```python
from build123d import *

# Parameters (mm, degrees)
BOSS_EXTRUDE4_DEPTH      = 20
SKETCH3_R                = 8.25
CUT_EXTRUDE1_DEPTH       = 7
CUT_EXTRUDE2_START       = -7
SKETCH4_R                = 8.25
CUT_EXTRUDE2_DEPTH       = 7
CUT_EXTRUDE3_DEPTH       = 128.220772675
SKETCH6_R                = 5
CUT_EXTRUDE4_DEPTH       = 16.6
FILLET1_R                = 3
BOSS_EXTRUDE5_DEPTH      = 20
BOSS_EXTRUDE6_DEPTH      = 46
BOSS_EXTRUDE6_DEPTH_BACK = 25
SKETCH8_R                = 11
SKETCH8_R_2              = 8.25
BOSS_EXTRUDE7_REACH      = 138.572
SKETCH9_W                = 20
SKETCH9_H                = 10
FILLET2_R                = 5
FILLET5_R                = 5
SKETCH10_W               = 60.25
SKETCH10_H               = 70.5
CUT_EXTRUDE5_DEPTH       = 128.619062056
BOSS_EXTRUDE8_DEPTH      = 20
BOSS_EXTRUDE9_START      = -20
SKETCH12_R               = 11
BOSS_EXTRUDE9_DEPTH      = 20
SKETCH13_OUTSIDE_W       = 202.602
SKETCH13_OUTSIDE_H       = 60.102
SKETCH13_OUTSIDE_W_2     = 164.5
SKETCH13_OUTSIDE_H_2     = 20
CUT_EXTRUDE6_DEPTH       = 152.565373684


with BuildPart() as part:
    # Sketch2 → Boss-Extrude4 (new body)
    with BuildSketch(Plane.XY):
        with BuildLine():
            Line((-100, 10.25), (0, 10.25))
            ThreePointArc((0, 10.25), (10.25, 0), (0, -10.25))
            Line((0, -10.25), (-100, -10.25))
            ThreePointArc((-100, -10.25), (-110.25, 0), (-100, 10.25))
        make_face()
        with BuildLine():
            Line((-7.247844507, -7.247844507), (-57.247844507, 42.752155493))
            ThreePointArc((-57.247844507, 42.752155493), (-57.247844507, 57.247844507), (-42.752155493, 57.247844507))
            Line((-42.752155493, 57.247844507), (7.247844507, 7.247844507))
            ThreePointArc((7.247844507, 7.247844507), (7.247844507, -7.247844507), (-7.247844507, -7.247844507))
        make_face()
        with BuildLine():
            Line((-107.247844507, 7.247844507), (-57.247844507, 57.247844507))
            ThreePointArc((-57.247844507, 57.247844507), (-42.752155493, 57.247844507), (-42.752155493, 42.752155493))
            Line((-42.752155493, 42.752155493), (-92.752155493, -7.247844507))
            ThreePointArc((-92.752155493, -7.247844507), (-107.247844507, -7.247844507), (-107.247844507, 7.247844507))
        make_face()
    extrude(amount=BOSS_EXTRUDE4_DEPTH)

    # Sketch3 → Cut-Extrude1 (cut)
    with BuildSketch(Plane(origin=(0, 0, 0), x_dir=(-1, 0, 0), z_dir=(0, 0, -1))):
        Circle(SKETCH3_R)
        with Locations((50, 50)):
            Circle(SKETCH3_R)
        with Locations((100, 0)):
            Circle(SKETCH3_R)
    extrude(amount=-CUT_EXTRUDE1_DEPTH, mode=Mode.SUBTRACT)

    # Sketch4 → Cut-Extrude2 (cut)
    with BuildSketch(Plane.XY.offset(20).offset(CUT_EXTRUDE2_START)):
        with Locations(Location((-100, 0, 0), (0, 0, 180))):
            Circle(SKETCH4_R)
        with Locations(Location((-50, 50, 0), (0, 0, 180))):
            Circle(SKETCH4_R)
        with Locations(Location((0, 0, 0), (0, 0, 180))):
            Circle(SKETCH4_R)
    extrude(amount=CUT_EXTRUDE2_DEPTH, mode=Mode.SUBTRACT)

    # Sketch5 → Cut-Extrude3 (cut, through all)
    with BuildSketch(Plane(origin=(0, 0, 0), x_dir=(-1, 0, 0), z_dir=(0, 0, -1))):
        Polygon((17.5, 8.25), (50, 40.75), (82.5, 8.25), align=None)
    extrude(amount=-CUT_EXTRUDE3_DEPTH, mode=Mode.SUBTRACT)

    # Sketch6 → Cut-Extrude4 (cut)
    with BuildSketch(Plane.XY.offset(20)):
        with Locations((-100, 0)):
            Circle(SKETCH6_R)
        with Locations((-50, 50)):
            Circle(SKETCH6_R)
        Circle(SKETCH6_R)
    extrude(amount=-CUT_EXTRUDE4_DEPTH, mode=Mode.SUBTRACT)

    # Fillet1
    fillet1_edges = [part.edges().sort_by_distance(p)[0] for p in [
        (-82.5, 8.25, 10),
        (-17.5, 8.25, 10),
        (-50, 40.75, 10),
    ]]
    fillet(fillet1_edges, radius=FILLET1_R)

    # Sketch7 → Boss-Extrude5 (add)
    with BuildSketch(Plane(origin=(0, 0, 0), x_dir=(-1, 0, 0), z_dir=(0, 0, -1))):
        with BuildLine():
            Line((-10.25, 14.75), (-10.25, 0))
            ThreePointArc((-10.25, 0), (-9.469765208, 3.922505182), (-7.247844507, 7.247844507))
            Line((-7.247844507, 7.247844507), (0.254310986, 14.75))
            Line((0.254310986, 14.75), (-10.25, 14.75))
        make_face()
        with BuildLine():
            Line((-10.25, -10.25), (0, -10.25))
            ThreePointArc((0, -10.25), (-7.247844507, -7.247844507), (-10.25, 0))
            Line((-10.25, 0), (-10.25, -10.25))
        make_face()
    extrude(amount=-BOSS_EXTRUDE5_DEPTH)

    # Sketch8 → Boss-Extrude6 (add, two sides: drawn at the far end of the back side and taken through both)
    # profile 1 of 3: a face of its own
    with BuildSketch(Plane(origin=(0, 14.75, 0), x_dir=(1, 0, 0), z_dir=(0, 1, 0)).offset(-BOSS_EXTRUDE6_DEPTH_BACK)):
        with BuildLine():
            Line((10.25, 0), (10.25, -10))
            ThreePointArc((10.25, -10), (13.110659193, -2.600599266), (20.204751131, 0.950226244))
            Line((20.204751131, 0.950226244), (10.25, 0))
        make_face()
    # profile 2 of 3: a face of its own
    with BuildSketch(Plane(origin=(0, 14.75, 0), x_dir=(1, 0, 0), z_dir=(0, 1, 0)).offset(-BOSS_EXTRUDE6_DEPTH_BACK)):
        with Locations((21.25, -10)):
            Circle(SKETCH8_R)
        with Locations(Location((21.25, -10, 0), (0, 0, 270))):
            Circle(SKETCH8_R_2, mode=Mode.SUBTRACT)
    # profile 3 of 3: a face of its own
    with BuildSketch(Plane(origin=(0, 14.75, 0), x_dir=(1, 0, 0), z_dir=(0, 1, 0)).offset(-BOSS_EXTRUDE6_DEPTH_BACK)):
        with BuildLine():
            Line((10.25, -10), (10.25, -20))
            Line((10.25, -20), (20.204751131, -20.950226244))
            ThreePointArc((20.204751131, -20.950226244), (13.110659193, -17.399400734), (10.25, -10))
        make_face()
    extrude(amount=BOSS_EXTRUDE6_DEPTH + BOSS_EXTRUDE6_DEPTH_BACK)

    # Boss-Extrude7: up to this plane
    boss_extrude7_end = Plane(origin=(7.247844507, 7.247844507, 20), z_dir=(-0.7071067811865439, -0.7071067811865512, 0))
    # Sketch9 → Boss-Extrude7 (add, up to the surface)
    with BuildSketch(Plane.ZY.offset(-10.25), mode=Mode.PRIVATE) as boss_extrude7_sk1:
        with Locations((10, 55.75)):
            Rectangle(SKETCH9_W, SKETCH9_H)
    boss_extrude7_tool1 = split(extrude(boss_extrude7_sk1.sketch, amount=BOSS_EXTRUDE7_REACH, mode=Mode.PRIVATE), bisect_by=boss_extrude7_end, keep=Keep.BOTH, mode=Mode.PRIVATE)
    add(boss_extrude7_tool1.solids().sort_by_distance((10.25, 55.75, 10))[0])

    # Fillet2
    # the kernel refuses this fillet: 5 mm, written as the material it adds along each edge
    with BuildSketch(Plane(origin=(10.25, 14.75, 0), x_dir=(-1, 0, 0), z_dir=(0, -1, 0)), Plane(origin=(10.25, -10.25, 20), x_dir=(-1, 0, 0), z_dir=(0, 1, 0))) as fillet2_piece_1:
        with BuildLine():
            CenterArc((FILLET2_R * 0.047619047619, FILLET2_R), FILLET2_R, 264.547378012, 5.452621988)
            Line((-FILLET2_R * 0.0474035768153, FILLET2_R * 0.00452488687783), (0, 0))
            Line((0, 0), (FILLET2_R * 0.047619047619, 0))
        make_face()
    extrude(amount=25)
    with BuildSketch(Plane(origin=(10.25, 50.75, 0), x_dir=(-1, 0, 0), z_dir=(0, 1, 0)), Plane(origin=(10.25, 60.75, 20), x_dir=(-1, 0, 0), z_dir=(0, -1, 0))) as fillet2_piece_2:
        with BuildLine():
            CenterArc((FILLET2_R * 0.047619047619, -FILLET2_R), FILLET2_R, 90, 5.452621988)
            Line((-FILLET2_R * 0.0474035768153, -FILLET2_R * 0.00452488687783), (0, 0))
            Line((0, 0), (FILLET2_R * 0.047619047619, 0))
        make_face()
    extrude(amount=10)

    # Fillet5
    fillet5_edges = [part.edges().sort_by_distance(p)[0] for p in [
        (-0.254310986, 14.75, 10),
        (-36.254310986, 50.75, 10),
    ]]
    fillet(fillet5_edges, radius=FILLET5_R)

    # Sketch10 → Cut-Extrude5 (cut, through all)
    with BuildSketch(Plane(origin=(0, 0, 0), x_dir=(-1, 0, 0), z_dir=(0, 0, -1))):
        with Locations((80.125, 25)):
            Rectangle(SKETCH10_W, SKETCH10_H)
    extrude(amount=-CUT_EXTRUDE5_DEPTH, mode=Mode.SUBTRACT)

    # Mirror1: part across plane


with BuildPart() as part_1:
    add(part.part)
    add(part.part.mirror(Plane(origin=(-50, -10.25, 21), x_dir=(0, 0, 1), z_dir=(1, 0, 0))))

    # Sketch11 → Boss-Extrude8 (add)
    with BuildSketch(Plane(origin=(0, 0, 0), x_dir=(-1, 0, 0), z_dir=(0, 0, -1))):
        with BuildLine():
            Line((46.254310986, 60.75), (53.745689014, 60.75))
            Line((53.745689014, 60.75), (57.247844507, 57.247844507))
            ThreePointArc((57.247844507, 57.247844507), (50, 60.25), (42.752155493, 57.247844507))
            Line((42.752155493, 57.247844507), (46.254310986, 60.75))
        make_face()
    extrude(amount=-BOSS_EXTRUDE8_DEPTH)

    # Sketch12 → Boss-Extrude9 (add)
    with BuildSketch(Plane(origin=(0, 60.75, 0), x_dir=(1, 0, 0), z_dir=(0, 1, 0)).offset(BOSS_EXTRUDE9_START)):
        with Locations((-121.25, -10)):
            Circle(SKETCH12_R)
        with Locations((21.25, -10)):
            Circle(SKETCH12_R)
    extrude(amount=BOSS_EXTRUDE9_DEPTH)

    # Sketch13 outside → Cut-Extrude6 (cut, through all)
    with BuildSketch(Plane(origin=(0, 60.75, 0), x_dir=(1, 0, 0), z_dir=(0, 1, 0))):
        with Locations((-50, -10)):
            Rectangle(SKETCH13_OUTSIDE_W, SKETCH13_OUTSIDE_H)
        with Locations((-50, -10)):
            Rectangle(SKETCH13_OUTSIDE_W_2, SKETCH13_OUTSIDE_H_2, mode=Mode.SUBTRACT)
    extrude(amount=-CUT_EXTRUDE6_DEPTH, mode=Mode.SUBTRACT)


solid = part_1.part
```
Work out the finished part from the listing and answer in its coordinate system (mm). A direction names the side the tool comes from. Round coordinates to 2 decimals unless told otherwise and drop trailing zeros. Loops run counter-clockwise (first coordinate to the right, second up) from the corner with the lowest first, then second, coordinate; pieces in that order, holes last.
(1) The mould has two halves that part along Y. Classify faces 1 (the flat face through (-51.1, 41.5, 0)), 2 (the flat face through (-64.93, 25.82, 9.86)), 3 (the flat face through (-49, 60.75, 10)): pulls with the +Y half, pulls with the -Y half, needs draft (parallel to the pull), parting line crosses it, or undercut.
Computed values:
face 1: needs draft
face 2: undercut
face 3: pulls with the +Y half
(2) The part is cut by section A-A, the plane y = 0. Give the number of separate pieces and of enclosed holes in the cut face, and give its area (3 significant figures).
Computed values:
separate pieces: 3
enclosed holes: 2
area: 2,210 mm2
(3) The part is cut by section B-B, the plane x = -50. Give the vertices of the cut face in (y, z), and give its area (3 significant figures).
Computed values:
outline: (-10.25, 0) - (8.25, 0) - (8.25, 20) - (-10.25, 20) - close; (39.51, 0) - (41.75, 0) - (41.75, 7) - (45, 7) - (45, 13) - (41.75, 13) - (41.75, 20) - (39.51, 20) - close; (55, 7) - (58.25, 7) - (58.25, 0) - (60.75, 0) - (60.75, 20) - (58.25, 20) - (58.25, 13) - (55, 13) - close
area: 504 mm2
(4) For faces 4 (the cylindrical face through (13.2, 14.9, 8.2)), 5 (the flat face through (-7, 50.75, 10)), 6 (the cylindrical face through (-7.87, -2.48, 16.45)), 7 (the cylindrical face through (-7.62, -3.16, 3.45)), determine the directions among +Z, -Z, +X, -X, +Y, -Y from which every point of the face is accessible in a straight line to the end or side of a thin tool.
Computed values:
face 4: -Y
face 5: +Z, -Z
face 6: +Z
face 7: -Z
(5) Each of these flat-tipped pins is pushed along its axis until it touches: P1, Ø5, axis at x = -124.5, z = 13.5, coming from the -Y side; P2, Ø5, axis at x = 4, y = -2, coming from the -Z side; P3, Ø6, axis at y = 40, z = 13, coming from the -X side; P4, Ø16, axis at x = -100, y = 0, coming from the +Z side. Where does it stop, or does it pass through?
Computed values:
P1: stops at y = 40.75
P2: stops at z = 7
P3: stops at x = -132.25
P4: stops at z = 13
(6) The part is cut by section D-D, the plane y = 24. Give the vertices of the cut face in (x, z), and give its area (3 significant figures).
Computed values:
outline: (-125.83, 0) - (-110.25, 0) - (-110.25, 20) - (-125.83, 20) arc R11 ccw to start; (-90.5, 0) - (-66.75, 0) - (-66.75, 20) - (-90.5, 20) - close; (-33.25, 0) - (-9.5, 0) - (-9.5, 20) - (-33.25, 20) - close; (10.25, 0) - (25.83, 0) arc R11 ccw to (25.83, 20) - (10.25, 20) - close; hole circle Ø16.5 at (-121.25, 10); hole circle Ø16.5 at (21.25, 10)
area: 1,330 mm2
(7) Find the intervals of material crossed by L1, parallel to Y at x = -50, z = 4; L2, parallel to Y at x = -50, z = 10.7; L3, parallel to Z at x = -121.25, y = 3, in increasing order.
Computed values:
L1: y = -10.25 to 8.25, 39.51 to 41.75, 58.25 to 60.75
L2: y = -10.25 to 8.25, 39.51 to 45, 55 to 60.75
L3: z = 0 to 1.75, 18.25 to 20
